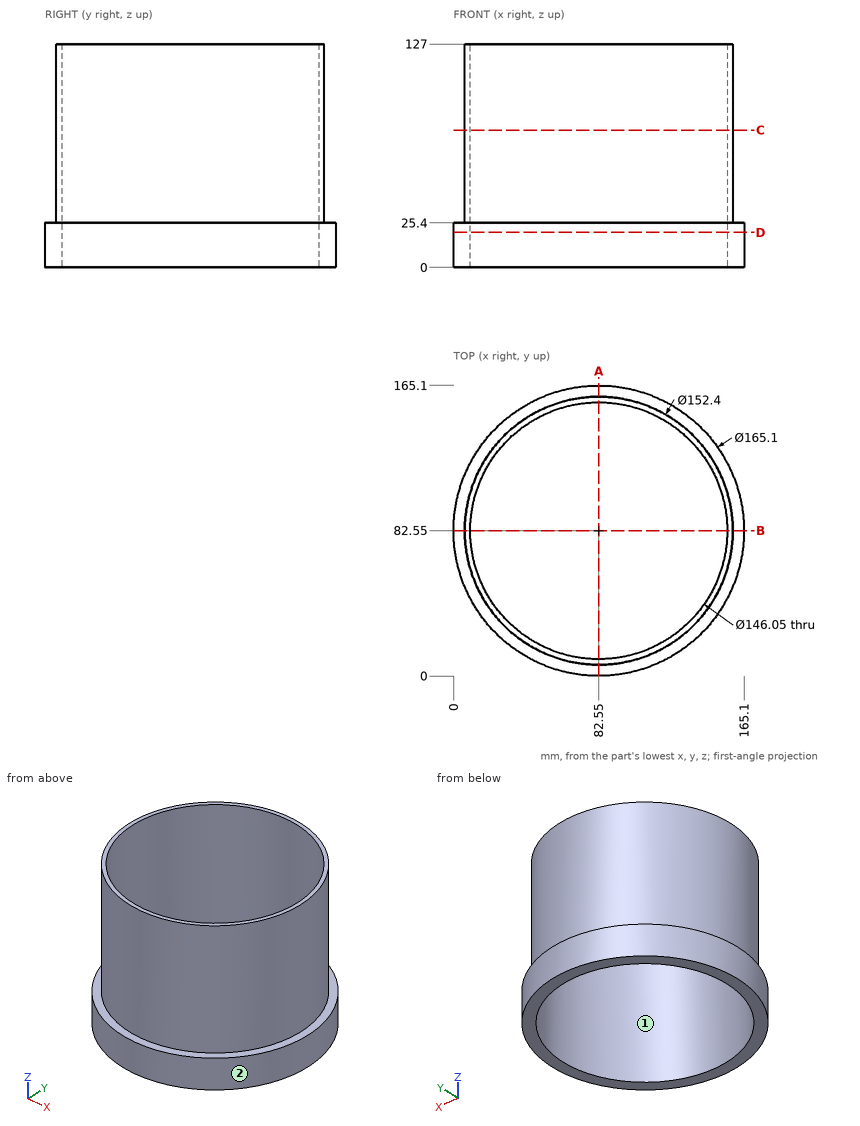
Can you work these out from the drawing? Everything is in mm from the part's minimum corner. Give positions to 0.01 mm unless a question says otherwise; leave off trailing zeros. Loops run counter-clockwise (first coordinate to the right, second up) from the corner with the lowest first, then second, coordinate; pieces in that order, holes last. Notation, with made-up numbers: M -35.75,51 L -27.75,51 A8 cw -27.75,63 Z; hole C 7.25,71.5 d10. An arc over 180 degrees is marked long. Put each result on its own line as item: value. Start each with the question number.
(1) I need wall thicknesses on line 1 along Y through (x, z) = (82, 89); line 2 along Y through (x, z) = (85, 75). Which ranges of each line are inside material? Lowest first, please. Write a range as [from, to].
(2) I want a section at A-A on x = 82.55. Please give me the cut outline in (y, z) (3 decimals).
(3) I want a section at D-D on z = 20. Please give me the cut outline in (x, y) (3 decimals).
(4) Will these pins go through, and if not, where does the flat tip stop? pin 1 Ø3 at (x, z) = (33, 87) entering from +Y; pin 2 Ø10 at (y, z) = (61, 74) entering from +X; pin 3 Ø8 at (x, z) = (69.5, 84) entering from -Y.
(5) If we mould it in two halves opening along X, with no side actions, what happens to the marked faces 1 and 2? For each: +X half, -X half, draft (parallel to the pull), parting line (faces both ways), or undercut.
(6) I want a section at C-C on z = 78. Please give me the cut outline in (x, y) (3 decimals), then the cut area to 3 significant figures.
Answer block:
1. line 1: [6.35, 9.53], [155.57, 158.75]
1. line 2: [6.39, 9.57], [155.53, 158.71]
2. outline: M 0,0 L 9.525,0 L 9.525,127 L 6.35,127 L 6.35,25.4 L 0,25.4 Z; M 155.575,0 L 165.1,0 L 165.1,25.4 L 158.75,25.4 L 158.75,127 L 155.575,127 Z
3. outline: C 82.55,82.55 d165.1; hole C 82.55,82.55 d146.05
4. pin 1: y = 141.69
4. pin 2: x = 156.93
4. pin 3: y = 6.89
5. face 1: undercut
5. face 2: parting line
6. outline: C 82.55,82.55 d152.4; hole C 82.55,82.55 d146.05
6. area: 1,490 mm^2
